from build123d import *

# Parameters (mm, degrees)
SKETCH_1_W      = 57
SKETCH_1_H      = 115
EXTRUDE_1_DEPTH = 8.5
FILLET_1_R      = 2
SKETCH_3_R      = 2.5


with BuildPart() as part:
    # 草图1 → 凸台-拉伸1 (new body, symmetric)
    with BuildSketch(Plane(origin=(0, 0, 0), x_dir=(1, 0, 0), z_dir=(0, 1, 0))):
        Rectangle(SKETCH_1_W, SKETCH_1_H)
    extrude(amount=EXTRUDE_1_DEPTH, both=True)

    # 圆角1
    fillet_1_edges = [part.edges().sort_by_distance(p)[0] for p in [
        (28.5, 8.5, 0),
        (0, 8.5, -57.5),
        (-28.5, 8.5, 0),
        (0, -8.5, -57.5),
        (28.5, -8.5, 0),
        (0, -8.5, 57.5),
        (-28.5, -8.5, 0),
        (0, 8.5, 57.5),
        (-28.5, 0, -57.5),
        (28.5, 0, -57.5),
        (28.5, 0, 57.5),
        (-28.5, 0, 57.5),
    ]]
    fillet(fillet_1_edges, radius=FILLET_1_R)

    # 扫描1: sweep along a path in 草图2
    with BuildLine(Plane(origin=(0, 0, 0), x_dir=(1, 0, 0), z_dir=(0, 1, 0))) as sweep_1_path:
        Line((-33, -12.5), (-33, -57.5))
        ThreePointArc((-33, -57.5), (-31.828427125, -60.328427125), (-29, -61.5))
        Line((-29, -61.5), (-4, -61.5))
        ThreePointArc((-4, -61.5), (-1.171572875, -60.328427125), (0, -57.5))
    # 草图3 → 扫描1 (sweep)
    with BuildSketch(Plane.XY.offset(57.5)):
        Circle(SKETCH_3_R)
    sweep(path=sweep_1_path.line)


solid = part.part
Verification items for the finished model (mm, model axes). A direction names the side the tool comes from. Coordinates: 2 decimals unless noted, no trailing zeros. Write each loop counter-clockwise with the first axis right and the second up, starting at its lowest first coordinate (ties: lowest second). Pieces come first, ordered by that corner, then holes. Notation, with made-up numbers: M -39,77.25 L 4,77.25 A22 ccw 4,100.25 Z; hole C 6.5,38.5 d2. An arc over 180 degrees is marked long. Use a Markdown table: item, result.
Q1. Sectioned sample at B-B, the plane y = 4.75. Record the boundary of the cut face in (x, z).
Reply:
| item | result |
|---|---|
| outline | M -28.5,-55.5 A2 ccw -26.5,-57.5 L 26.5,-57.5 A2 ccw 28.5,-55.5 L 28.5,55.5 A2 ccw 26.5,57.5 L -26.5,57.5 A2 ccw -28.5,55.5 Z |
Q2. Set-up check for faces 1 (the face through (28.5, 0, 1)), 2 (the face through (-33, 0, 12.5)), 3 (the face through (-28.5, 0, 1)): record each of +Z, -Z, +X, -X, +Y, -Y from which the full face is reachable in a straight line by a thin tool's end or side.
Reply:
| item | result |
|---|---|
| face 1 | +Z, -Z, +X, +Y, -Y |
| face 2 | -Z, -X, +Y, -Y |
| face 3 | -Z, +Y, -Y |
Q3. Sectioned sample at C-C, the plane x = -10.5. Record the boundary of the cut face in (y, z), plus the area to 3 significant figures.
Reply:
| item | result |
|---|---|
| outline | M -8.5,-55.5 A2 ccw -6.5,-57.5 L 6.5,-57.5 A2 ccw 8.5,-55.5 L 8.5,55.5 A2 ccw 6.5,57.5 L -6.5,57.5 A2 ccw -8.5,55.5 Z; C 0,61.5 d5 |
| area | 1,970 mm² |
Q4. Sectioned sample at D-D, the plane z = 4.5. Record the boundary of the cut face in (x, y).
Reply:
| item | result |
|---|---|
| outline | M -28.5,-6.5 A2 ccw -26.5,-8.5 L 26.5,-8.5 A2 ccw 28.5,-6.5 L 28.5,6.5 A2 ccw 26.5,8.5 L -26.5,8.5 A2 ccw -28.5,6.5 Z |
Q5. Sectioned sample at A-A, the plane z = 30. Record the boundary of the cut face in (x, y).
Reply:
| item | result |
|---|---|
| outline | C -33,0 d5; M -28.5,-6.5 A2 ccw -26.5,-8.5 L 26.5,-8.5 A2 ccw 28.5,-6.5 L 28.5,6.5 A2 ccw 26.5,8.5 L -26.5,8.5 A2 ccw -28.5,6.5 Z |
Q6. Go/stop test with flat-tipped pins: P1, Ø10, axis at y = -3.5, z = -3.5, coming from the -X side; P2, Ø5.5, axis at x = -34, y = -1, coming from the -Z side. Record where each tip stops, or that it passes through.
Reply:
| item | result |
|---|---|
| P1 | stops at x = -28.5 |
| P2 | stops at z = 12.5 |
Q7. Thickness scan on line 1 (X direction, y = 1, z = 2.5); line 2 (Z direction, x = -14.5, y = -4.25); line 3 (Z direction, x = -21, y = 1). Record the ranges inside material, lowest first.
Reply:
| item | result |
|---|---|
| line 1 | x = -28.5 to 28.5 |
| line 2 | z = -57.5 to 57.5 |
| line 3 | z = -57.5 to 57.5, 59.21 to 63.79 |
Q8. Draft check along Z on faces 4 (the face through (-16.32, 0.96, 63.81)), 5 (the face through (0, 0, -57.5)), 6 (the face through (-35.31, 0.96, 35.32)). Enter one of: +Z half, -Z half, draft (parallel to the pull), parting line (faces both ways), or undercut.
Reply:
| item | result |
|---|---|
| face 4 | undercut |
| face 5 | -Z half |
| face 6 | draft |
